```python
from build123d import *

# Parameters (mm, degrees)
BOSS_EXTRUDE1_DEPTH = 4
CUT_EXTRUDE1_REACH  = 149.251
SKETCH2_W           = 32
SKETCH2_H           = 37
SKETCH3_W           = 32
SKETCH3_H           = 44
CUT_EXTRUDE2_DEPTH  = 1.2
BOSS_EXTRUDE2_DEPTH = 3
CUT_EXTRUDE3_REACH  = 149.251
SKETCH5_W           = 80
SKETCH5_H           = 2
SKETCH13_W          = 10
SKETCH13_H          = 17
BOSS_EXTRUDE3_DEPTH = 6.5
LPATTERN1_COUNT     = 2
LPATTERN1_PITCH     = 6.8
CHAMFER1_SIZE       = 6
CHAMFER1_SIZE2      = 5.034597787
FILLET1_R           = 2


with BuildPart() as part:
    # Sketch1 → Boss-Extrude1 (new body)
    with BuildSketch(Plane(origin=(0, 0, 0), x_dir=(1, 0, 0), z_dir=(0, 1, 0))):
        with BuildLine():
            Line((-40, 68), (-40, 120))
            Line((-40, 120), (-46.677171015, 131.565199449))
            ThreePointArc((-46.677171015, 131.565199449), (0, 139.6), (46.677171015, 131.565199449))
            Line((46.677171015, 131.565199449), (40, 120))
            Line((40, 120), (40, 68))
            Line((40, 68), (-40, 68))
        make_face()
    extrude(amount=BOSS_EXTRUDE1_DEPTH)

    # Sketch2 → Cut-Extrude1 (cut, up to next)
    with BuildSketch(Plane(origin=(0, 4, 0), x_dir=(1, 0, 0), z_dir=(0, 1, 0)), mode=Mode.PRIVATE) as cut_extrude1_sk1:
        with Locations((5, 93.5)):
            Rectangle(SKETCH2_W, SKETCH2_H)
    cut_extrude1_tool1 = extrude(cut_extrude1_sk1.sketch, amount=-CUT_EXTRUDE1_REACH, mode=Mode.PRIVATE) & part.part
    add(cut_extrude1_tool1.solids().sort_by_distance((5, 4, -93.5))[0], mode=Mode.SUBTRACT)

    # Sketch3 → Cut-Extrude2 (cut)
    with BuildSketch(Plane.XZ):
        with Locations((5, -93.5)):
            Rectangle(SKETCH3_W, SKETCH3_H)
    extrude(amount=-CUT_EXTRUDE2_DEPTH, mode=Mode.SUBTRACT)

    # Sketch4 → Boss-Extrude2 (add)
    with BuildSketch(Plane.XZ):
        with BuildLine():
            Line((-40, -78), (-40, -130.236102159))
            ThreePointArc((-40, -130.236102159), (0, -136.240384268), (40, -130.236102159))
            Line((40, -130.236102159), (40, -78))
            Line((40, -78), (37, -78))
            Line((37, -78), (37, -128))
            ThreePointArc((37, -128), (0, -133.240384268), (-37, -128))
            Line((-37, -128), (-37, -78))
            Line((-37, -78), (-40, -78))
        make_face()
    extrude(amount=BOSS_EXTRUDE2_DEPTH)

    # Sketch5 → Cut-Extrude3 (cut, up to next)
    with BuildSketch(Plane.XZ, mode=Mode.PRIVATE) as cut_extrude3_sk1:
        with Locations((0, -69)):
            Rectangle(SKETCH5_W, SKETCH5_H)
    cut_extrude3_tool1 = extrude(cut_extrude3_sk1.sketch, amount=-CUT_EXTRUDE3_REACH, mode=Mode.PRIVATE) & part.part
    add(cut_extrude3_tool1.solids().sort_by_distance((0, 0, -69))[0], mode=Mode.SUBTRACT)

    # Sketch13 → Boss-Extrude3 (add)
    with BuildSketch(Plane.XZ):
        with Locations((-16, -109)):
            Rectangle(SKETCH13_W, SKETCH13_H)
    extrude(amount=BOSS_EXTRUDE3_DEPTH)

    # Cut-Loft1: read off the stored shape, not the designer's step
    # Cut-Loft1: loft between two sections, ruled curve by curve
    cut_loft1_from = [
        Edge.make_bspline([(-18.5, 4, -108.3), (-19.001373519, 4, -108.3), (-20.004120556, 4, -108.3), (-20.723714816, 4, -108.3), (-21.292720218, 4, -108.3), (-21.789967148, 4, -108.441885809), (-22.316617117, 4, -108.86202161), (-22.630245954, 4, -109.404072839), (-22.73490999, 4, -110), (-22.630245954, 4, -110.595927161), (-22.316617117, 4, -111.13797839), (-21.789967148, 4, -111.558114191), (-21.292720218, 4, -111.7), (-20.723714816, 4, -111.7), (-20.004120556, 4, -111.7), (-18.5, 4, -111.7), (-16.995879444, 4, -111.7), (-16.276285184, 4, -111.7), (-15.707279782, 4, -111.7), (-15.210032852, 4, -111.558114191), (-14.683382883, 4, -111.13797839), (-14.369754046, 4, -110.595927161), (-14.26509001, 4, -110), (-14.369754046, 4, -109.404072839), (-14.683382883, 4, -108.86202161), (-15.210032852, 4, -108.441885809), (-15.707279782, 4, -108.3), (-16.276285184, 4, -108.3), (-16.995879444, 4, -108.3), (-17.998626481, 4, -108.3), (-18.5, 4, -108.3)], [0.419845373, 0.419845373, 0.419845373, 0.419845373, 0.459922687, 0.5, 0.5, 0.542461343, 0.584922687, 0.62738403, 0.669845373, 0.712306716, 0.75476806, 0.797229403, 0.839690746, 0.839690746, 0.87976806, 0.919845373, 0.959922687, 1, 1, 1.042461343, 1.084922687, 1.12738403, 1.169845373, 1.212306716, 1.25476806, 1.297229403, 1.339690746, 1.339690746, 1.37976806, 1.419845373, 1.419845373, 1.419845373, 1.419845373], 3),
    ]
    cut_loft1_to = [
        Edge.make_bspline([(-12.7, -6.5, -111.8), (-12.771947826, -6.5, -111.8), (-12.915843478, -6.5, -111.8), (-13.030587652, -6.5, -111.8), (-13.379489971, -6.5, -111.8), (-13.760605324, -6.5, -111.856871893), (-14.332360426, -6.5, -112.171543481), (-14.782964502, -6.5, -112.74231317), (-14.958930975, -6.5, -113.5), (-14.782964502, -6.5, -114.25768683), (-14.332360426, -6.5, -114.828456519), (-13.760605324, -6.5, -115.143128107), (-13.379489971, -6.5, -115.2), (-13.030587652, -6.5, -115.2), (-12.915843478, -6.5, -115.2), (-12.7, -6.5, -115.2), (-12.484156522, -6.5, -115.2), (-12.369412348, -6.5, -115.2), (-12.020510029, -6.5, -115.2), (-11.639394676, -6.5, -115.143128107), (-11.067639574, -6.5, -114.828456519), (-10.617035498, -6.5, -114.25768683), (-10.441069025, -6.5, -113.5), (-10.617035498, -6.5, -112.74231317), (-11.067639574, -6.5, -112.171543481), (-11.639394676, -6.5, -111.856871893), (-12.020510029, -6.5, -111.8), (-12.369412348, -6.5, -111.8), (-12.484156522, -6.5, -111.8), (-12.628052174, -6.5, -111.8), (-12.7, -6.5, -111.8)], [0.419845373, 0.419845373, 0.419845373, 0.419845373, 0.459922687, 0.5, 0.5, 0.542461343, 0.584922687, 0.62738403, 0.669845373, 0.712306716, 0.75476806, 0.797229403, 0.839690746, 0.839690746, 0.87976806, 0.919845373, 0.959922687, 1, 1, 1.042461343, 1.084922687, 1.12738403, 1.169845373, 1.212306716, 1.25476806, 1.297229403, 1.339690746, 1.339690746, 1.37976806, 1.419845373, 1.419845373, 1.419845373, 1.419845373], 3),
    ]
    cut_loft1 = Solid(Shell([*[Face.make_surface_from_curves(cut_loft1_from[k], cut_loft1_to[k]) for k in range(1)], Face(Wire(cut_loft1_from)), Face(Wire(cut_loft1_to))]))
    add(cut_loft1, mode=Mode.SUBTRACT)

    # LPattern1: Cut-Loft1 ×2
    with Locations(*[(0, 0, i * LPATTERN1_PITCH) for i in range(1, LPATTERN1_COUNT)]):
        add(cut_loft1, mode=Mode.SUBTRACT)

    # Chamfer1
    chamfer1_edges = [part.edges().sort_by_distance(p)[0] for p in [
        (-21, -6.5, -109),
    ]]
    chamfer1_side = [part.faces().sort_by_distance(p)[0] for p in [
        (-21, -3.25, -109),
    ]]
    chamfer(chamfer1_edges, length=CHAMFER1_SIZE, length2=CHAMFER1_SIZE2, reference=chamfer1_side[0])

    # Fillet1
    fillet1_edges = [part.edges().sort_by_distance(p)[0] for p in [
        (-18.482701106, -3.5, -100.5),
        (-18.482701106, -3.5, -117.5),
        (-11, -3.25, -117.5),
        (-11, -3.25, -100.5),
    ]]
    fillet(fillet1_edges, radius=FILLET1_R)


solid = part.part
```
Verification items for the finished model (mm, model axes). A direction names the side the tool comes from. Round coordinates to 2 decimals unless told otherwise and drop trailing zeros. Write each loop counter-clockwise with the first axis right and the second up, starting at its lowest first coordinate (ties: lowest second). Pieces come first, ordered by that corner, then holes.
1. Section check A-A on z = -89. Enter the section's corners in (x, y), plus the area to 3 significant figures.
2. Scan lines: L1, parallel to X at y = -2.75, z = -101; L2, parallel to X at y = -0.25, z = -100; L3, parallel to X at y = -2.5, z = -104.5. Record each from-to range of solid material in increasing order.
3. Access from +Z, -Z, +X, -X, +Y, -Y to the whole of each face (thin tool, end or side, straight path). Record for faces 1 (the cylindrical face through (-11.6, -3.3, -101.07)), 2 (the flat face through (0.2, 0, -136.4)), 3 (the flat face through (5, 1.2, -73)), 4 (the flat face through (-38, -1, -78)).
4. Section check B-B on x = 16. Enter the section's corners in (y, z).
5. Section check C-C on x = 33.5. Enter the section's corners in (y, z), plus the area to 3 significant figures.
6. Gauge pin test, flat ends, axial feed: P1, Ø1.5, axis at y = -3.5, z = -101.5, coming from the -X side; P2, Ø3.5, axis at y = 0.5, z = -102.5, coming from the +X side; P3, Ø1.5, axis at x = 38, y = -1.5, coming from the +Z side; P4, Ø1, axis at x = 14.5, y = -4, coming from the +Z side. Record the tip position at first contact, or that the pin passes through.
7. Section check D-D on z = -124. Enter the section's corners in (x, y).
8. Draft check along Z on faces 5 (the cylindrical face through (-0.57, -1.48, -136.24)), 6 (the flat face through (43.385, 1.972, -125.864)), 7 (the flat face through (-15, -2, -117.5)), 8 (the flat face through (-18.45, -3.54, -109.09)). Enter one of: +Z half, -Z half, draft (parallel to the pull), parting line (faces both ways), or undercut.
Answer:
1. outline: (-40, -3) - (-37, -3) - (-37, 0) - (-11, 0) - (-11, 4) - (-40, 4) - close; (21, 0) - (37, 0) - (37, -3) - (40, -3) - (40, 4) - (21, 4) - close
1. area: 210 mm2
2. L1: x = -40 to -37, -18.23 to -11.68, 37 to 40
2. L2: x = -40 to -37, 37 to 40
2. L3: x = -40 to -37, -19.32 to -17.63, -12.19 to -11, 37 to 40
3. face 1: +Z, -Y
3. face 2: -Z, -Y
3. face 3: -Y
3. face 4: +Z, +X, -X, -Y
4. outline: (-3, -135.3) - (0, -135.3) - (0, -138.68) - (4, -138.68) - (4, -112) - (1.2, -112) - (1.2, -115.5) - (0, -115.5) - (0, -132.28) - (-3, -132.28) - close; (0, -71.5) - (1.2, -71.5) - (1.2, -75) - (4, -75) - (4, -70) - (0, -70) - close
5. outline: (-3, -132.06) - (0, -132.06) - (0, -135.52) - (4, -135.52) - (4, -70) - (0, -70) - (0, -128.96) - (-3, -128.96) - close
5. area: 271 mm2
6. P1: stops at x = -40
6. P2: stops at x = 40
6. P3: stops at z = -78
6. P4: passes through
7. outline: (-42.31, 0) - (-40, 0) - (-40, -3) - (-37, -3) - (-37, 0) - (37, 0) - (37, -3) - (40, -3) - (40, 0) - (42.31, 0) - (42.31, 4) - (-42.31, 4) - close
8. face 5: -Z half
8. face 6: +Z half
8. face 7: undercut
8. face 8: draft
